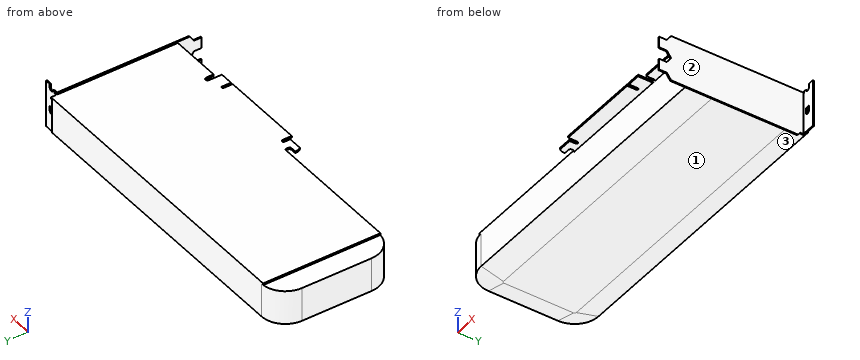
from build123d import *

# Parameters (mm, degrees)
F1_DEPTH  = 1.5
F3_DEPTH  = 1
F4_R      = 0.99999
F5_R      = 1.74999
F6_R      = 1.24999
F7_R      = 1.5
F9_DEPTH  = 1
F11_DEPTH = 33.5
F12_SIZE2 = 5
F12_SIZE  = 18.6602540378


# Not quite as in the source:
# - a fillet or chamfer is up to 0.001 mm smaller than in the source, because OpenCascade refuses the exact size


with BuildPart() as f1:
    # F0 (on Top) → F1 (new body)
    with BuildSketch(Plane.XY):
        Polygon((84.5, -53.25), (127.5, -53.25), (127.5, 53.25), (-127.5, 53.25), (-127.5, -45.25), (-12.5, -45.25), (-12.5, -49.75), (-18.5, -49.75), (-18.5, -52.25), (-17, -54.75), (-5.5, -54.75), (-5.5, -48.75), (-3, -48.75), (-3, -57.75), (68, -57.75), (68, -49.25), (70, -49.25), (70, -57.75), (81, -57.75), (81, -45.25), (84.5, -45.25), align=None)
    extrude(amount=F1_DEPTH)

    # F2 (on face) → F3 (join)
    with BuildSketch(Plane.YZ.offset(127.5)):
        Polygon((47.75, 2.5), (-63.25, 2.5), (-66.75, -2.5), (-73.25, -2.5), (-73.25, -11.75), (-66.75, -11.75), (-63.25, -16.75), (-66.75, -21.75), (-73.25, -21.75), (-73.25, -31), (-66.75, -31), (-63.25, -36), (43.25, -36), (45.25, -33.5), (47.75, -33.5), align=None)
    extrude(amount=F3_DEPTH)

    # F4 (radius 1 in the source; OpenCascade refuses exactly that, so slightly less here)
    f4_edges = [f1.edges().sort_by_distance(p)[0] for p in [
        (68, -49.25, 0.75),
        (70, -49.25, 0.75),
    ]]
    fillet(f4_edges, radius=F4_R)

    # F5 (radius 1.75 in the source; OpenCascade refuses exactly that, so slightly less here)
    f5_edges = [f1.edges().sort_by_distance(p)[0] for p in [
        (81, -45.25, 0.75),
        (84.5, -45.25, 0.75),
    ]]
    fillet(f5_edges, radius=F5_R)

    # F6 (radius 1.25 in the source; OpenCascade refuses exactly that, so slightly less here)
    f6_edges = [f1.edges().sort_by_distance(p)[0] for p in [
        (-5.5, -48.75, 0.75),
        (-3, -48.75, 0.75),
    ]]
    fillet(f6_edges, radius=F6_R)

    # F7
    f7_edges = [f1.edges().sort_by_distance(p)[0] for p in [
        (-12.5, -49.75, 0.75),
        (-12.5, -45.25, 0.75),
    ]]
    fillet(f7_edges, radius=F7_R)

    # F8 (on face) → F9 (join)
    with BuildSketch(Plane(origin=(0, 47.75, 0), x_dir=(-1, 0, 0), z_dir=(0, 1, 0))):
        with BuildLine():
            Line((-140, -33.5), (-127.5, -33.5))
            Line((-127.5, -33.5), (-127.5, 1.5))
            Line((-127.5, 1.5), (-129.5, 1.5))
            Line((-129.5, 1.5), (-129.5, 3))
            Line((-129.5, 3), (-131.5, 3))
            ThreePointArc((-131.5, 3), (-133.5, 1), (-135.5, 3))
            Line((-135.5, 3), (-135.5, 6))
            Line((-135.5, 6), (-140, 6))
            Line((-140, 6), (-140, -33.5))
        make_face()
        with BuildLine():
            Line((-135.5, -17), (-135.5, -13))
            Line((-135.5, -13), (-131.5, -13))
            Line((-131.5, -13), (-131.5, -17))
            ThreePointArc((-131.5, -17), (-133.5, -19), (-135.5, -17))
        make_face(mode=Mode.SUBTRACT)
    extrude(amount=F9_DEPTH)

    # F10 (on face) → F11 (join, through all)
    with BuildSketch(Plane(origin=(0, 0, 0), x_dir=(1, 0, 0), z_dir=(0, 0, -1))):
        with BuildLine():
            Line((126.5, -53.25), (126.5, 45.25))
            Line((126.5, 45.25), (-125.5, 45.25))
            ThreePointArc((-125.5, 45.25), (-139.6421356237, 39.3921356237), (-145.5, 25.25))
            Line((-145.5, 25.25), (-145.5, -33.25))
            ThreePointArc((-145.5, -33.25), (-139.6421356237, -47.3921356237), (-125.5, -53.25))
            Line((-125.5, -53.25), (126.5, -53.25))
        make_face()
    extrude(amount=F11_DEPTH)

    # F12
    f12_edges = [f1.edges().sort_by_distance(p)[0] for p in [
        (0.5, -45.25, -33.5),
        (0.5, 53.25, -33.5),
    ]]
    f12_side = f1.faces().sort_by_distance((-8.651711, 4, -33.5))[0]
    chamfer(f12_edges, length=F12_SIZE, length2=F12_SIZE2, reference=f12_side)


solid = f1.part
Check sheet for the modelled part. Datum: model origin and axes. Units: mm. Face numbers are marked on the shaded views. A direction names the side the tool comes from. Give positions to 0.01 mm unless a question says otherwise; leave off trailing zeros. Loops run counter-clockwise (first coordinate to the right, second up) from the corner with the lowest first, then second, coordinate; pieces in that order, holes last. Notation, with made-up numbers: M 43.5,-10.75 L 90.5,-10.75 A13 cw 90.5,9.25 Z; hole C -3,60 d9. An arc over 180 degrees is marked long. Return JSON: item names as keys, results as strings. Group by question number.
1. Cross-section at B-B on x = -40. Record the boundary of the cut face in (y, z).
2. Tool access check on the marked faces 1, 2 and 3. Record the directions out of +Z, -Z, +X, -X, +Y, -Y that give a thin tool (end or side, any length) a straight path to the whole face; none if there is none.
3. Cross-section at A-A on y = -21. Record the boundary of the cut face in (x, z), plus the area to 3 significant figures.
4. Thickness scan on L1, parallel to Y at x = 109.5, z = -4; L2, parallel to Z at x = -88.5, y = -5; L3, parallel to X at y = -55, z = -26. Record the ranges inside material, lowest first.
5. Go/stop test with flat-tipped pins: pin 1 (1.1 mm diameter, centred on x = 128, z = 2, fed in from +Y); pin 2 (17 mm diameter, centred on y = 19, z = -12.5, fed in from +X); pin 3 (1.6 mm diameter, centred on x = 28, z = 0.5, fed in from -Y). Record where each tip stops, or that it passes through.
Return value:
{
 "1": {"outline": "M -45.25,-28.5 L -26.59,-33.5 L 34.59,-33.5 L 53.25,-28.5 L 53.25,1.5 L -45.25,1.5 Z"},
 "2": {"face 1": "-Z, -X, +Y, -Y", "face 2": "+Z, -Z, +X, -Y", "face 3": "-Z, -X, +Y"},
 "3": {"outline": "M -145.5,-28.5 L -126.84,-33.5 L 126.5,-33.5 L 126.5,0 L 127.5,0 L 127.5,-36 L 128.5,-36 L 128.5,2.5 L 127.5,2.5 L 127.5,1.5 L -127.5,1.5 L -127.5,0 L -145.5,0 Z", "area": "9,490 mm^2"},
 "4": {"L1": "-45.25 to 53.25", "L2": "-33.5 to 1.5", "L3": "127.5 to 128.5"},
 "5": {"pin 1": "y = 48.75", "pin 2": "x = 128.5", "pin 3": "y = -57.75"}
}
